Verification items for the finished model (mm, model axes). A direction names the side the tool comes from. Give positions to 0.01 mm unless a question says otherwise; leave off trailing zeros. Loops run counter-clockwise (first coordinate to the right, second up) from the corner with the lowest first, then second, coordinate; pieces in that order, holes last. Notation, with made-up numbers: (24, -7) - (41, -7) arc R8 ccw to (41, 1) - close; hole circle Ø10 at (1.25, 11). An arc over 180 degrees is marked (long way). One line per item, written item: value. Start each with the question number.
1. Sectioned sample at D-D (y = 1.75). Record the cut outline in (x, z), plus the area to 3 significant figures.
2. Scan lines: L1, parallel to X at y = 1.4, z = -12.7; L2, parallel to Y at x = -24.1, z = -12.7. Record each from-to range of solid material in increasing order. Write a range as [from, to].
3. Access from +Z, -Z, +X, -X, +Y, -Y to the whole of each face (thin tool, end or side, straight path). Record for faces 4 (the flat face through (-17, 2, 0)), 5 (the flat face through (-8, 3.175, -13)).
4. Sectioned sample at A-A (y = 12.7). Record the cut outline in (x, z) (3 decimals).
5. Mould release check, pull along Z, two halves, no side actions. Record for faces 1 (the cylindrical face through (-13.474, 1.61, -9.216)), 2 (the flat face through (-15.34, 0, -15.34)), 3 (the flat face through (-23, 7, -25.4)): pulls with the +Z half, pulls with the -Z half, needs draft (parallel to the pull), parting line crosses it, or undercut.
6. Sectioned sample at C-C (x = -12.7). Record the cut outline in (y, z) (3 decimals), plus the area to 3 significant figures.
7. Sectioned sample at B-B (z = -12.7). Record the cut outline in (x, y) (3 decimals).
8. Gauge pin test, flat ends, axial feed: pin 1 (4 mm diameter, centred on x = -12, z = -6.5, fed in from -Y); pin 2 (11.5 mm diameter, centred on y = 12.7, z = -12.7, fed in from +X) (3 decimals); pin 3 (10 mm diameter, centred on x = -11.5, y = 10, fed in from +Z); pin 4 (9.5 mm diameter, centred on x = -12.7, z = -12.7, fed in from +Y) (3 decimals). Record the tip position at first contact, or that the pin passes through.
Autodesk Inventor part; units mm, degrees
ref_plane "YZ Plane" through (0, 0, 0) normal (1, 0, 0) x (0, 1, 0)
ref_plane "XZ Plane" through (0, 0, 0) normal (0, 1, 0) x (-1, 0, 0)
ref_plane "XY Plane" through (0, 0, 0) normal (0, 0, 1) x (1, 0, 0)
sketch "Sketch1" plane through (0, 0, 0) normal (0, 1, 0) x (-1, 0, 0)
  line L0 (0, 0) -> (25.4, 0)
  line L1 (25.4, 0) -> (25.4, -25.4)
  line L2 (25.4, -25.4) -> (0, -25.4)
  line L3 (0, -25.4) -> (0, 0)
  dimension "d0" = 25.4
  dimension "d1" = 25.4
extrude "Extrusion1" add sketch "Sketch1" along normal blind 3.175
sketch "Sketch2" plane through (0, 3.175, 0) normal (0, 1, 0) x (1, 0, 0)
  line L0 (-25.4, 25.4) -> (-25.4, 0)
  line L1 (-25.4, 0) -> (-22.225, 0)
  line L2 (-22.225, 0) -> (-22.225, 25.4)
  line L3 (-22.225, 25.4) -> (-25.4, 25.4)
  line L4 (-25.4, 25.4) -> (-25.4, 0)
  point P0 (0, 0)
  dimension "d4" = 3.175
  dimension "d5" = 25.4
extrude "Extrusion2" add sketch "Sketch2" along normal blind 22.225
sketch "Sketch3" plane through (0, 3.175, 0) normal (0, 1, 0) x (1, 0, 0)
  circle A0 centre (-12.7, 12.7) radius 3.5687
  line L0 (0, 25.4) -> (-22.225, 25.4)
  line L1 (0, 25.4) -> (0, 0)
  dimension "d8" = 7.1374
  dimension "d9" = 12.7
  dimension "d10" = 12.7
extrude "Extrusion3" cut sketch "Sketch3" against normal blind 22.225
sketch "Sketch4" plane through (-22.225, 3.175, 0) normal (1, 0, 0) x (0, 0, -1)
  circle A0 centre (12.7, 9.525) radius 3.5687
  line L0 (25.4, 0) -> (25.4, 22.225)
  line L1 (0, 22.225) -> (25.4, 22.225)
  point P0 (0, -3.175)
  dimension "d13" = 7.1374
  dimension "d14" = 12.7
  dimension "d15" = 12.7
extrude "Extrusion4" cut sketch "Sketch4" against normal blind 3.175
properties part number "Lbracket" material "Aluminum 6061"
Results are:
1. outline: (-25.4, -25.4) - (0, -25.4) - (0, 0) - (-25.4, 0) - close; hole circle Ø7.14 at (-12.7, -12.7)
1. area: 605 mm^2
2. L1: x = [-25.4, -16.27], [-9.13, 0]
2. L2: y = [0, 9.13], [16.27, 25.4]
3. face 4: +Z, +X, -X, +Y, -Y
3. face 5: +Z, -Z, +X, +Y
4. outline: (-25.4, -25.4) - (-22.225, -25.4) - (-22.225, -16.269) - (-25.4, -16.269) - close; (-25.4, -9.131) - (-22.225, -9.131) - (-22.225, 0) - (-25.4, 0) - close
5. face 1: undercut
5. face 2: needs draft
5. face 3: pulls with the -Z half
6. outline: (0, -25.4) - (3.175, -25.4) - (3.175, -16.269) - (0, -16.269) - close; (0, -9.131) - (3.175, -9.131) - (3.175, 0) - (0, 0) - close
6. area: 58.0 mm^2
7. outline: (-25.4, 0) - (-16.269, 0) - (-16.269, 3.175) - (-22.225, 3.175) - (-22.225, 9.131) - (-25.4, 9.131) - close; (-25.4, 16.269) - (-22.225, 16.269) - (-22.225, 25.4) - (-25.4, 25.4) - close; (-9.131, 0) - (0, 0) - (0, 3.175) - (-9.131, 3.175) - close
8. pin 1: stops at y = 0
8. pin 2: stops at x = -22.225
8. pin 3: passes through
8. pin 4: stops at y = 3.175
